from build123d import *

# Parameters (mm, degrees)
SKETCH_2_R          = 2
EXTRUDE_1_DEPTH     = 31
EXTRUDE_1_2_DEPTH   = 31
EXTRUDE_1_3_DEPTH   = 31
EXTRUDE_1_4_DEPTH   = 31
SKETCH_3_W          = 81
SKETCH_3_H          = 101
EXTRUDE_2_DEPTH     = 31
EXTRUDE_3_DEPTH     = 2
CUT_EXTRUDE_1_REACH = 86
SKETCH_5_W          = 8
SKETCH_5_H          = 22
CUT_EXTRUDE_2_REACH = 86
SKETCH_6_W          = 5.5
SKETCH_6_H          = 13
CUT_EXTRUDE_3_REACH = 106
SKETCH_7_W          = 13
SKETCH_7_H          = 5
SKETCH_8_R          = 3
EXTRUDE_4_DEPTH     = 5
SKETCH_9_R          = 2
CUT_EXTRUDE_4_DEPTH = 5
SKETCH_10_W         = 80
SKETCH_10_H         = 12
EXTRUDE_5_DEPTH     = 5
SKETCH_11_W         = 3
SKETCH_11_H         = 11.8
EXTRUDE_6_DEPTH     = 80
CUT_EXTRUDE_5_DEPTH = 3
SKETCH_13_R         = 1.6
CUT_EXTRUDE_6_DEPTH = 3
SKETCH_14_W         = 31
SKETCH_14_H         = 1
EXTRUDE_7_DEPTH     = 3
SKETCH_15_W         = 31
SKETCH_15_H         = 1
EXTRUDE_8_DEPTH     = 3


with BuildPart() as part:
    # Sketch 2 → Extrude 1 (new body)
    with BuildSketch(Plane.XY):
        with BuildLine():
            Line((-38.968626967, -45.5), (-40.968626967, -45.5))
            Line((-40.968626967, -45.5), (-40.968626967, -44.5))
            Line((-40.968626967, -44.5), (-38.968626967, -44.5))
            ThreePointArc((-38.968626967, -44.5), (-32.171572875, -42.171572875), (-34.5, -48.968626967))
            Line((-34.5, -48.968626967), (-34.5, -50.968626967))
            Line((-34.5, -50.968626967), (-35.5, -50.968626967))
            Line((-35.5, -50.968626967), (-35.5, -48.968626967))
            ThreePointArc((-35.5, -48.968626967), (-37.828427125, -47.828427125), (-38.968626967, -45.5))
        make_face()
        with Locations((-35, -45)):
            Circle(SKETCH_2_R, mode=Mode.SUBTRACT)
    extrude(amount=-EXTRUDE_1_DEPTH)



with BuildPart() as body_2:
    # Sketch 2 → Extrude 1 2 (new body)
    with BuildSketch(Plane.XY):
        with BuildLine():
            Line((-35.5, 50.968626967), (-34.5, 50.968626967))
            Line((-34.5, 50.968626967), (-34.5, 48.968626967))
            ThreePointArc((-34.5, 48.968626967), (-32.171572875, 42.171572875), (-38.968626967, 44.5))
            Line((-38.968626967, 44.5), (-40.968626967, 44.5))
            Line((-40.968626967, 44.5), (-40.968626967, 45.5))
            Line((-40.968626967, 45.5), (-38.968626967, 45.5))
            ThreePointArc((-38.968626967, 45.5), (-37.828427125, 47.828427125), (-35.5, 48.968626967))
            Line((-35.5, 48.968626967), (-35.5, 50.968626967))
        make_face()
        with Locations((-35, 45)):
            Circle(SKETCH_2_R, mode=Mode.SUBTRACT)
    extrude(amount=-EXTRUDE_1_2_DEPTH)


with BuildPart() as body_3:
    # Sketch 2 → Extrude 1 3 (new body)
    with BuildSketch(Plane.XY):
        with BuildLine():
            Line((34.5, 50.968626967), (35.5, 50.968626967))
            Line((35.5, 50.968626967), (35.5, 48.968626967))
            ThreePointArc((35.5, 48.968626967), (37.828427125, 47.828427125), (38.968626967, 45.5))
            Line((38.968626967, 45.5), (40.968626967, 45.5))
            Line((40.968626967, 45.5), (40.968626967, 44.5))
            Line((40.968626967, 44.5), (38.968626967, 44.5))
            ThreePointArc((38.968626967, 44.5), (32.171572875, 42.171572875), (34.5, 48.968626967))
            Line((34.5, 48.968626967), (34.5, 50.968626967))
        make_face()
        with Locations((35, 45)):
            Circle(SKETCH_2_R, mode=Mode.SUBTRACT)
    extrude(amount=-EXTRUDE_1_3_DEPTH)


with BuildPart() as body_4:
    # Sketch 2 → Extrude 1 4 (new body)
    with BuildSketch(Plane.XY):
        with BuildLine():
            Line((40.602402736, -44.5), (40.602402736, -45.5))
            Line((40.602402736, -45.5), (37.602402736, -45.5))
            ThreePointArc((37.602402736, -45.5), (36.87383297, -46.87383297), (35.5, -47.602402736))
            Line((35.5, -47.602402736), (35.5, -50.602402736))
            Line((35.5, -50.602402736), (34.5, -50.602402736))
            Line((34.5, -50.602402736), (34.5, -47.602402736))
            ThreePointArc((34.5, -47.602402736), (33.12616703, -43.12616703), (37.602402736, -44.5))
            Line((37.602402736, -44.5), (40.602402736, -44.5))
        make_face()
        with Locations((35, -45)):
            Circle(SKETCH_2_R, mode=Mode.SUBTRACT)
    extrude(amount=-EXTRUDE_1_4_DEPTH)


with BuildPart() as body_5:
    # Sketch 3 → Extrude 2 (new body)
    with BuildSketch(Plane(origin=(0, 0, -31), x_dir=(-1, 0, 0), z_dir=(0, 0, -1))):
        with BuildLine():
            Line((-40, -52), (40, -52))
            ThreePointArc((40, -52), (41.414213562, -51.414213562), (42, -50))
            Line((42, -50), (42, 50))
            ThreePointArc((42, 50), (41.414213562, 51.414213562), (40, 52))
            Line((40, 52), (-40, 52))
            ThreePointArc((-40, 52), (-41.414213562, 51.414213562), (-42, 50))
            Line((-42, 50), (-42, -50))
            ThreePointArc((-42, -50), (-41.414213562, -51.414213562), (-40, -52))
        make_face()
        Rectangle(SKETCH_3_W, SKETCH_3_H, mode=Mode.SUBTRACT)
    extrude(amount=-EXTRUDE_2_DEPTH)


with BuildPart() as part_1:
    add(part.part)

    add(body_2.part)  # Extrude 3 merges body 2

    add(body_3.part)  # Extrude 3 merges body 3

    add(body_4.part)  # Extrude 3 merges body 4

    add(body_5.part)  # Extrude 3 merges body 5
    # Sketch 4 → Extrude 3 (add)
    with BuildSketch(Plane(origin=(0, 0, -31), x_dir=(-1, 0, 0), z_dir=(0, 0, -1))):
        with BuildLine():
            Line((40, 52), (-40, 52))
            ThreePointArc((-40, 52), (-41.414213562, 51.414213562), (-42, 50))
            Line((-42, 50), (-42, -50))
            ThreePointArc((-42, -50), (-41.414213562, -51.414213562), (-40, -52))
            Line((-40, -52), (40, -52))
            ThreePointArc((40, -52), (41.414213562, -51.414213562), (42, -50))
            Line((42, -50), (42, 50))
            ThreePointArc((42, 50), (41.414213562, 51.414213562), (40, 52))
        make_face()
    extrude(amount=EXTRUDE_3_DEPTH)

    # Sketch 5 → Cut-Extrude 1 (cut, up to next)
    with BuildSketch(Plane.ZY.offset(42), mode=Mode.PRIVATE) as cut_extrude_1_sk1:
        with Locations((-4, 0.5)):
            Rectangle(SKETCH_5_W, SKETCH_5_H)
    cut_extrude_1_tool1 = extrude(cut_extrude_1_sk1.sketch, amount=-CUT_EXTRUDE_1_REACH, mode=Mode.PRIVATE) & part_1.part
    add(cut_extrude_1_tool1.solids().sort_by_distance((-42, 0.5, -4))[0], mode=Mode.SUBTRACT)

    # Sketch 6 → Cut-Extrude 2 (cut, up to next)
    with BuildSketch(Plane(origin=(42, 0, 0), x_dir=(0, 0, -1), z_dir=(1, 0, 0)), mode=Mode.PRIVATE) as cut_extrude_2_sk1:
        with Locations((2.75, 0)):
            Rectangle(SKETCH_6_W, SKETCH_6_H)
    cut_extrude_2_tool1 = extrude(cut_extrude_2_sk1.sketch, amount=-CUT_EXTRUDE_2_REACH, mode=Mode.PRIVATE) & part_1.part
    add(cut_extrude_2_tool1.solids().sort_by_distance((42, 0, -2.75))[0], mode=Mode.SUBTRACT)

    # Sketch 7 → Cut-Extrude 3 (cut, up to next)
    with BuildSketch(Plane.XZ.offset(52), mode=Mode.PRIVATE) as cut_extrude_3_sk1:
        with BuildLine():
            Line((-2.213, -3.2), (-7.313, -3.2))
            ThreePointArc((-7.313, -3.2), (-9.313, -1.2), (-7.313, 0.8))
            Line((-7.313, 0.8), (-2.213, 0.8))
            ThreePointArc((-2.213, 0.8), (-0.213, -1.2), (-2.213, -3.2))
        make_face()
    cut_extrude_3_tool1 = extrude(cut_extrude_3_sk1.sketch, amount=-CUT_EXTRUDE_3_REACH, mode=Mode.PRIVATE) & part_1.part
    add(cut_extrude_3_tool1.solids().sort_by_distance((-4.763, -52, -1.2))[0], mode=Mode.SUBTRACT)
    # Sketch 7 → Cut-Extrude 3 (cut, up to next)
    with BuildSketch(Plane.XZ.offset(52), mode=Mode.PRIVATE) as cut_extrude_3_sk2:
        with Locations((9.397, -2.5)):
            Rectangle(SKETCH_7_W, SKETCH_7_H)
    cut_extrude_3_tool2 = extrude(cut_extrude_3_sk2.sketch, amount=-CUT_EXTRUDE_3_REACH, mode=Mode.PRIVATE) & part_1.part
    add(cut_extrude_3_tool2.solids().sort_by_distance((9.397, -52, -2.5))[0], mode=Mode.SUBTRACT)

    # Sketch 8 → Extrude 4 (add)
    with BuildSketch(Plane.XY.offset(-31)):
        with Locations((-15, -34.5)):
            Circle(SKETCH_8_R)
        with Locations((15, -34.5)):
            Circle(SKETCH_8_R)
        with Locations((-10, 46)):
            Circle(SKETCH_8_R)
        with Locations((10, 46)):
            Circle(SKETCH_8_R)
        with Locations((-10, 30)):
            Circle(SKETCH_8_R)
        with Locations((10, 30)):
            Circle(SKETCH_8_R)
    extrude(amount=EXTRUDE_4_DEPTH)

    # Sketch 9 → Cut-Extrude 4 (cut)
    with BuildSketch(Plane(origin=(0, 0, -33), x_dir=(-1, 0, 0), z_dir=(0, 0, -1))):
        with Locations((-15, -34.5)):
            Circle(SKETCH_9_R)
        with Locations((15, -34.5)):
            Circle(SKETCH_9_R)
        with Locations((-10, 46)):
            Circle(SKETCH_9_R)
        with Locations((10, 46)):
            Circle(SKETCH_9_R)
        with Locations((10, 30)):
            Circle(SKETCH_9_R)
        with Locations((-10, 30)):
            Circle(SKETCH_9_R)
    extrude(amount=-CUT_EXTRUDE_4_DEPTH, mode=Mode.SUBTRACT)

    # Sketch 10 → Extrude 5 (add)
    with BuildSketch(Plane(origin=(0, 52, 0), x_dir=(1, 0, 0), z_dir=(0, 1, 0))):
        with Locations((0, 27)):
            Rectangle(SKETCH_10_W, SKETCH_10_H)
    extrude(amount=EXTRUDE_5_DEPTH)

    # Sketch 11 → Extrude 6 (add)
    with BuildSketch(Plane.ZY.offset(40)):
        Polygon((-33, 57), (-33, 68.8), (-29.3, 68.8), (-29.3, 64), (-31, 62.3), (-31, 57), align=None)
        with Locations((-22.5, 62.9)):
            Rectangle(SKETCH_11_W, SKETCH_11_H)
    extrude(amount=-EXTRUDE_6_DEPTH)

    # Sketch 12 → Cut-Extrude 5 (cut)
    with BuildSketch(Plane(origin=(0, 0, -24), x_dir=(-1, 0, 0), z_dir=(0, 0, -1))):
        with BuildLine():
            Line((-35, 61.2), (35, 61.2))
            ThreePointArc((35, 61.2), (36.2, 60), (35, 58.8))
            Line((35, 58.8), (-35, 58.8))
            ThreePointArc((-35, 58.8), (-36.2, 60), (-35, 61.2))
        make_face()
    extrude(amount=-CUT_EXTRUDE_5_DEPTH, mode=Mode.SUBTRACT)

    # Sketch 13 → Cut-Extrude 6 (cut, through all)
    with BuildSketch(Plane.XY.offset(-31)):
        with Locations((-31.5, -0.5)):
            Circle(SKETCH_13_R)
        with Locations((31.5, -0.5)):
            Circle(SKETCH_13_R)
    extrude(amount=-CUT_EXTRUDE_6_DEPTH, mode=Mode.SUBTRACT)

    # Sketch 14 → Extrude 7 (add)
    with BuildSketch(Plane(origin=(-40.5, 0, 0), x_dir=(0, 0, -1), z_dir=(1, 0, 0))):
        with Locations((15.5, 12)):
            Rectangle(SKETCH_14_W, SKETCH_14_H)
        with Locations((15.5, -11)):
            Rectangle(SKETCH_14_W, SKETCH_14_H)
    extrude(amount=EXTRUDE_7_DEPTH)

    # Sketch 15 → Extrude 8 (add)
    with BuildSketch(Plane.ZY.offset(-40.5)):
        with Locations((-15.5, 12)):
            Rectangle(SKETCH_15_W, SKETCH_15_H)
        with Locations((-15.5, -11)):
            Rectangle(SKETCH_15_W, SKETCH_15_H)
    extrude(amount=EXTRUDE_8_DEPTH)


solid = part_1.part
Verification items for the finished model (mm, model axes). A direction names the side the tool comes from. Coordinates: 2 decimals unless noted, no trailing zeros. Write each loop counter-clockwise with the first axis right and the second up, starting at its lowest first coordinate (ties: lowest second). Pieces come first, ordered by that corner, then holes. Notation, with made-up numbers: (71, 30.5) -> (122, 30.5) arc R23 ccw to (122, 52.5) -> close; hole circle Ø11 at (-2.5, 88). An arc over 180 degrees is marked (long way). One line per item, written item: value. Start each with the question number.
Q1. Access from +Z, -Z, +X, -X, +Y, -Y to the whole of each face (thin tool, end or side, straight path). Record for faces 1 (the flat face through (-1, 68.8, -31)), 2 (the cylindrical face through (10, 44, -31)), 3 (the flat face through (40, 56.8, -26.9)), 4 (the cylindrical face through (32.261, 42.085, -15.283)).
Q2. Cross-section at D-D on y = 20.5. Enter the section's corners in (x, z), and give its area (3 significant figures).
Q3. Cross-section at C-C on z = -14. State how many separate pieces and enclosed holes the cut face has, and give its area (3 significant figures).
Q4. Thickness scan on L1, parallel to Y at x = -10, z = -32; L2, parallel to X at y = -20, z = -17; L3, parallel to Y at x = -6, z = -6.5. Record the ranges inside material, lowest first. Write a range as from..to.
Q5. Go/stop test with flat-tipped pins: P1, Ø12, axis at x = 22, y = -21.5, coming from the +Z side; P2, Ø0.9, axis at x = 38.5, z = -18, coming from the +Y side; P3, Ø4.5, axis at x = -35, y = 44, coming from the +Z side; P4, Ø1.4, axis at x = -2, y = 66, coming from the +Z side. Record where each tip stops, or that it passes through.
Q6. Cross-section at A-A on x = 19.5. Enter the section's corners in (y, z), and give its area (3 significant figures).
Q7. Cross-section at B-B on y = -8.5. Enter the section's corners in (x, z).
Q8. Mould release check, pull along Y, two halves, no side actions. Record for faces 5 (the flat face through (1, -52, -16)), 6 (the cylindrical face through (-10, 49, -29)), 7 (the cylindrical face through (29.9, -0.43, -31.99)), 8 (the flat face through (-1, 52, -10)): pulls with the +Y half, pulls with the -Y half, needs draft (parallel to the pull), parting line crosses it, or undercut.
Checked values:
1. face 1: +Z, -Z, +X, -X, +Y
1. face 2: -Z
1. face 3: +Z, -Z, +X, +Y
1. face 4: +Z
2. outline: (-42, -33) -> (42, -33) -> (42, 0) -> (40.5, 0) -> (40.5, -31) -> (-40.5, -31) -> (-40.5, 0) -> (-42, 0) -> close
2. area: 261 mm²
3. separate pieces: 1
3. enclosed holes: 9
3. area: 701 mm²
4. L1: y = -52..28, 32..44, 48..68.8
4. L2: x = -42..-40.5, 40.5..42
4. L3: y = -52..-50.5, 50.5..52
5. P1: stops at z = -31
5. P2: stops at y = 52
5. P3: stops at z = 0
5. P4: stops at z = -21
6. outline: (-52, -33) -> (68.8, -33) -> (68.8, -29.3) -> (64, -29.3) -> (62.3, -31) -> (57, -31) -> (57, -24) -> (58.8, -24) -> (58.8, -21) -> (52, -21) -> (52, 0) -> (50.5, 0) -> (50.5, -31) -> (-50.5, -31) -> (-50.5, 0) -> (-52, 0) -> close; (61.2, -24) -> (68.8, -24) -> (68.8, -21) -> (61.2, -21) -> close
6. area: 422 mm²
7. outline: (-42, -33) -> (42, -33) -> (42, 0) -> (40.5, 0) -> (40.5, -31) -> (-40.5, -31) -> (-40.5, -8) -> (-42, -8) -> close
8. face 5: pulls with the -Y half
8. face 6: undercut
8. face 7: undercut
8. face 8: pulls with the +Y half
